Design review of the part built by this model. Coordinates are the model's own, in mm. Round coordinates to 2 decimals unless told otherwise and drop trailing zeros. Order: outer loops, then holes, each group sorted by start corner. A loop starts at its lowest first (then second) coordinate and runs counter-clockwise, first axis right, second up. Notation, with made-up numbers: M -2,-8 L 30,-8 A15 ccw 30,19 Z; hole C 78,4.25 d4. An arc over 180 degrees is marked long. Use a Markdown table: item, result. Add a question column.
(1) To check wall thickness, follow probe 1 along Z at (x, y) = (0, -1.2); probe 2 along Z at (x, y) = (0, -0.35); probe 3 along X at (y, z) = (174, 11.5). State the ranges of each line that lie inside material, in increasing order. Write a range as from..to.
(2) The part is to be moulded in two halves that separate along Y. For faces 1 (the face through (8.195, -99.753, -7.022)), 2 (the face through (0, -2, -22)), 3 (the face through (0, 0, -22)), say which applies: released by +Y, released by -Y, zero draft, split by the parting line, or undercut.
(3) Take a section at A-A (x = 0). Write out the cut boundary in (y, z), then the cut area to 3 significant figures.
(4) For pin 1 (8 mm diameter, centred on x = -3.5, y = 344, fed in from -Z); pin 2 (1.5 mm diameter, centred on x = -7, y = 98, fed in from -Z); pin 3 (4 mm diameter, centred on y = 454, z = 25, fed in from +X), all flat-tipped, find the tip position at first contact; note any pin that passes through.
Solid Edge part; units mm, degrees
sketch "Sketch1" plane through (2.3093, -0.1611, 2.3037) normal (0, 0.9976, 0.0698) x (1, 0, 0)
  circle A0 centre (-2.3093, 2.3093) radius 10
extrude "ExtrudedProtrusion_2" add sketch "Sketch1" against normal blind 100 and the other way blind 520
shell "Thinwall_2" thickness 2 removed faces 2 at (-6.4667, -99.2774, -13.8256) at (-6.4667, 519.2123, 29.4235)
sketch "Sketch2" plane through (0, 0, 0) normal (0, -1, 0) x (1, 0, 0)
  line L0 (10, -35) -> (-10, -35)
  line L1 (-10, -35) -> (-10, 0)
  line L2 (-10, 0) -> (10, 0)
  line L3 (10, 0) -> (10, -35)
extrude "ExtrudedProtrusion_3" add sketch "Sketch2" along normal blind 2
hole "Hole_1" at (0, -2, -28.57) direction (0, 1, 0) diameter 8 end up to next
properties material "Aluminum, 1060"
Verdict:
| question | item | result |
|---|---|---|
| 1 | probe 1 | z = -35..-32.57, -24.57..0, 7.94..9.94 |
| 1 | probe 2 | z = -35..-32.57, -24.57..0, 8..10 |
| 1 | probe 3 | x = -9.98..-7.97, 7.97..9.98 |
| 2 | face 1 | released by -Y |
| 2 | face 2 | undercut |
| 2 | face 3 | released by +Y |
| 3 | outline | M -100.45,3 L -100.31,1 L 518.18,44.25 L 518.04,46.25 Z; M -99.2,-14.96 L -99.06,-16.95 L -2,-10.16 L -2,-24.57 L 0,-24.57 L 0,-10.02 L 519.43,26.3 L 519.29,28.29 L 0,-8.02 L 0,0 L -2,0 L -2,-8.16 Z; M -2,-35 L 0,-35 L 0,-32.57 L -2,-32.57 Z |
| 3 | area | 2,530 mm^2 |
| 4 | pin 1 | stops at z = 13.86 |
| 4 | pin 2 | stops at z = -0.97 |
| 4 | pin 3 | stops at x = 8.81 |
